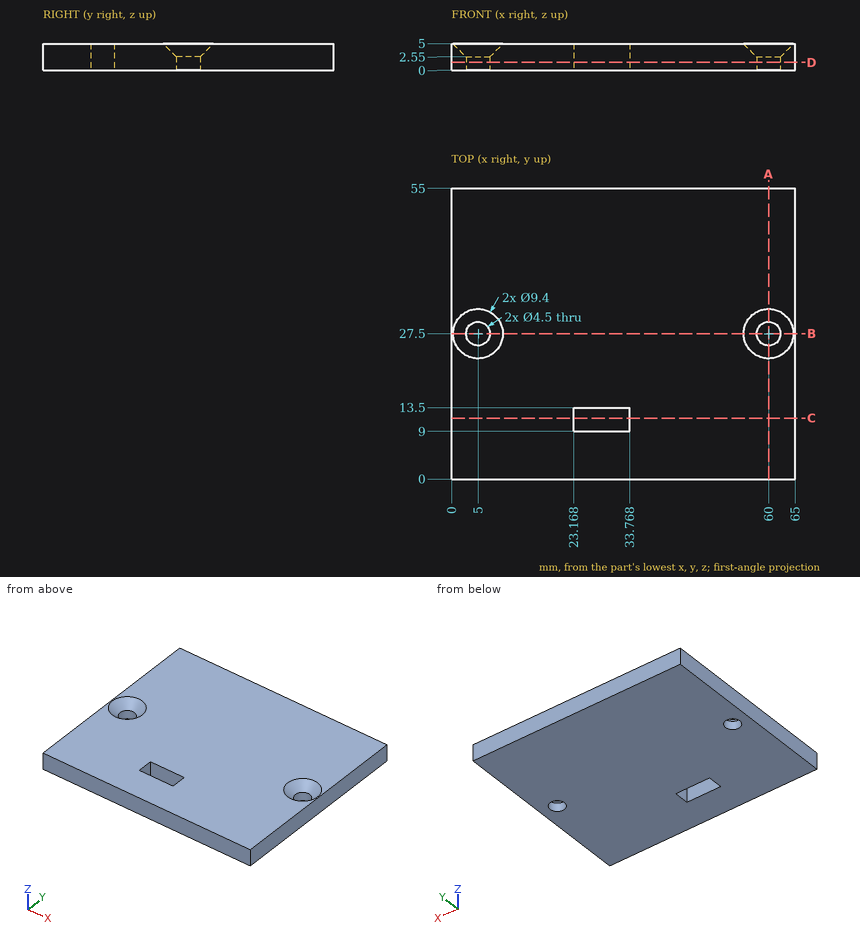
Answer from the drawing. Dimensions are ordinates in mm from the lowest x, y and z of the part. Give positions to 0.01 mm unless a question says otherwise; leave off trailing zeros. Loops run counter-clockwise (first coordinate to the right, second up) from the corner with the lowest first, then second, coordinate; pieces in that order, holes last. Notation, with made-up numbers: M -1,-39 L 17,-39 A28 cw 17,-4 Z; hole C -36,-35.5 d2. An arc over 180 degrees is marked long. One line per item, written item: value.
Q1. A flat-ended cylindrical pin translates along its axis: P1, Ø2, axis at y = 11, z = 1.5, coming from the -X side. Find the tip coordinate at first contact, or state that the pin passes through.
Working result:
P1: stops at x = 0
Q2. A cutting plane is placed at C-C on y = 11.5. Determine the outline of the cut face in (x, z).
Working result:
outline: M 0,0 L 23.17,0 L 23.17,5 L 0,5 Z; M 33.77,0 L 65,0 L 65,5 L 33.77,5 Z
Q3. A cutting plane is placed at A-A on x = 60. Determine the outline of the cut face in (y, z).
Working result:
outline: M 0,0 L 25.25,0 L 25.25,2.55 L 22.8,5 L 0,5 Z; M 29.75,0 L 55,0 L 55,5 L 32.2,5 L 29.75,2.55 Z
Q4. A cutting plane is placed at B-B on y = 27.5. Determine the outline of the cut face in (x, z), then the cut area to 3 significant figures.
Working result:
outline: M 0,0 L 2.75,0 L 2.75,2.55 L 0.3,5 L 0,5 Z; M 7.25,0 L 57.75,0 L 57.75,2.55 L 55.3,5 L 9.7,5 L 7.25,2.55 Z; M 62.25,0 L 65,0 L 65,5 L 64.7,5 L 62.25,2.55 Z
area: 268 mm^2
Q5. A cutting plane is placed at D-D on z = 1.5. Determine the outline of the cut face in (x, y), then the cut area to 3 significant figures.
Working result:
outline: M 0,0 L 65,0 L 65,55 L 0,55 Z; hole C 5,27.5 d4.5; hole M 23.17,9 L 33.77,9 L 33.77,13.5 L 23.17,13.5 Z; hole C 60,27.5 d4.5
area: 3,500 mm^2
Q6. Find the intervals of material crossed by line 1 (X direction, y = 27.5, z = 1.55); line 2 (Y direction, x = 60, z = 1.2); line 3 (X direction, y = 31, z = 4.2) (1 decimal), in increasing order. Write a range as from..to.
Working result:
line 1: x = 0..2.75, 7.25..57.75, 62.25..65
line 2: y = 0..25.25, 29.75..55
line 3: x = 0..3.3, 6.7..58.3, 61.7..65
